Check sheet for the drawn part. Datum: minimum x, y, z corner. Units: mm. Give positions to 0.01 mm unless a question says otherwise; leave off trailing zeros. Loops run counter-clockwise (first coordinate to the right, second up) from the corner with the lowest first, then second, coordinate; pieces in that order, holes last. Notation, with made-up numbers: M 47.25,-10 L 57.25,-10 A16 ccw 57.25,5 Z; hole C 71,-30.75 d8. An arc over 180 degrees is marked long. Write each question's results on one line, items separated by ' | '. Start each with the question number.
1. Sectioned sample at A-A on z = 2.45. Record the cut outline in (x, y).
2. Go/stop test with flat-tipped pins: pin 1 (3 mm diameter, centred on y = 11.5, z = 1.5, fed in from -X); pin 2 (1.2 mm diameter, centred on x = 31.5, z = 4.5, fed in from -Y); pin 3 (7.5 mm diameter, centred on x = 11.5, y = 29.5, fed in from +Z). Record where each tip stops, or that it passes through.
3. Material ranges on line 1 along Z through (x, y) = (47, 35); line 2 along Y through (x, z) = (45.5, 4.1); line 3 along Y through (x, z) = (31, 2.45), recorded low to high.
4. Draft check along Y on the marked faces 1, 2 and 3. Enter one of: pulls with the +Y half, pulls with the -Y half, needs draft (parallel to the pull), parting line crosses it, or undercut.
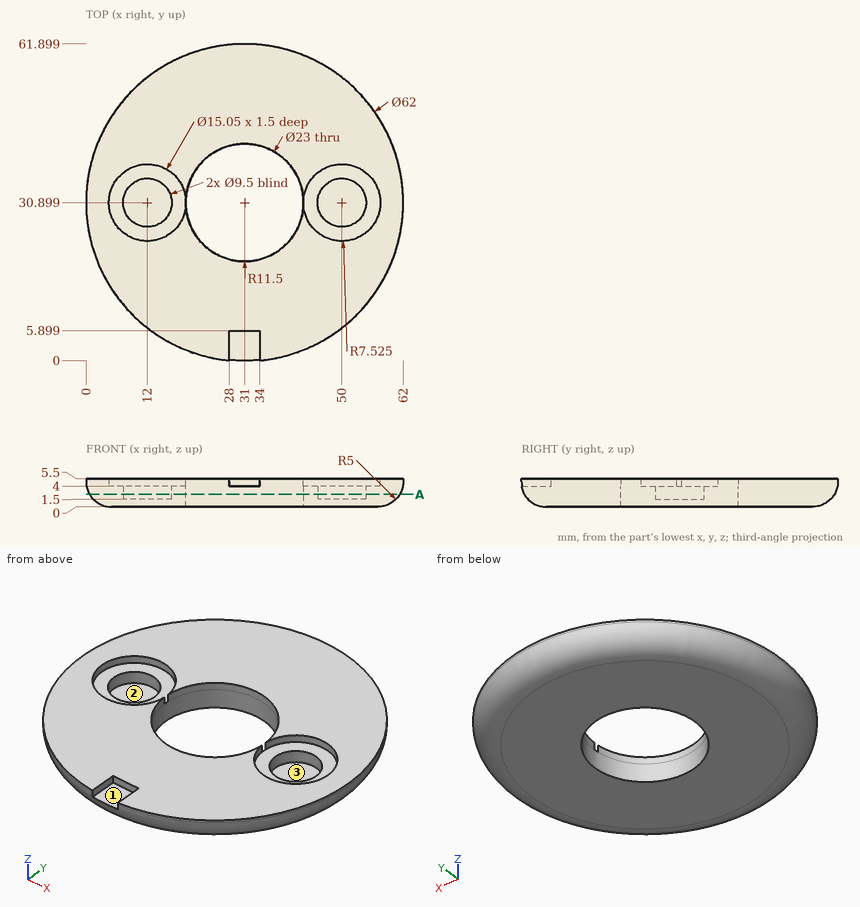
Output values:
1) outline: C 31,30.9 d60.6; hole C 12,30.9 d9.5; hole C 31,30.9 d23; hole C 50,30.9 d9.5
2) pin 1: x = 6.8 | pin 2: y = 0 | pin 3: z = 4
3) line 1: 0 to 4 | line 2: 3.59 to 24.87, 36.93 to 58.21 | line 3: 0.6 to 19.4, 42.4 to 61.2
4) face 1: needs draft | face 2: undercut | face 3: undercut
